Geometry check sheet. Reference: the model listing, model coordinates, mm. Face numbers are marked on the shaded views. A direction names the side the tool comes from. Coordinates: 2 decimals unless noted, no trailing zeros. Loops run counter-clockwise (first coordinate to the right, second up) from the corner with the lowest first, then second, coordinate; pieces in that order, holes last. Notation, with made-up numbers: (-9.5, 55.5) - (8.5, 55.5) arc R34 cw to (8.5, 85.5) - close; hole circle Ø5 at (34.25, -25). An arc over 180 degrees is marked (long way). One line per item, written item: value.
from build123d import *

# Parameters (mm, degrees)
SKETCH1_W                = 18.66
SKETCH1_H                = 2.314
BOSS_EXTRUDE1_DEPTH      = 2.6
BOSS_EXTRUDE2_DEPTH      = 3.91
BOSS_EXTRUDE2_DEPTH_BACK = 10.37
SKETCH2_R                = 0.33


with BuildPart() as part:
    # Sketch1 → Boss-Extrude1 (new body)
    with BuildSketch(Plane(origin=(0, 0, 0), x_dir=(1, 0, 0), z_dir=(0, 1, 0))):
        with Locations((9.33, 1.157)):
            Rectangle(SKETCH1_W, SKETCH1_H)
    extrude(amount=BOSS_EXTRUDE1_DEPTH)

    # Sketch2 → Boss-Extrude2 (add, two sides: drawn at the far end of the back side and taken through both)
    with BuildSketch(Plane(origin=(0, 2.6, 0), x_dir=(1, 0, 0), z_dir=(0, 1, 0)).offset(-BOSS_EXTRUDE2_DEPTH_BACK)):
        with Locations(Location((1.33, 1.157, 0), (0, 0, 270))):
            Circle(SKETCH2_R)
        with Locations(Location((3.11, 1.157, 0), (0, 0, 270))):
            Circle(SKETCH2_R)
        with Locations(Location((4.89, 1.157, 0), (0, 0, 270))):
            Circle(SKETCH2_R)
        with Locations(Location((6.67, 1.157, 0), (0, 0, 270))):
            Circle(SKETCH2_R)
        with Locations(Location((8.45, 1.157, 0), (0, 0, 270))):
            Circle(SKETCH2_R)
        with Locations(Location((10.23, 1.157, 0), (0, 0, 270))):
            Circle(SKETCH2_R)
        with Locations(Location((12.01, 1.157, 0), (0, 0, 270))):
            Circle(SKETCH2_R)
        with Locations(Location((13.79, 1.157, 0), (0, 0, 270))):
            Circle(SKETCH2_R)
        with Locations(Location((15.57, 1.157, 0), (0, 0, 270))):
            Circle(SKETCH2_R)
        with Locations(Location((17.35, 1.157, 0), (0, 0, 270))):
            Circle(SKETCH2_R)
    extrude(amount=BOSS_EXTRUDE2_DEPTH + BOSS_EXTRUDE2_DEPTH_BACK)


solid = part.part
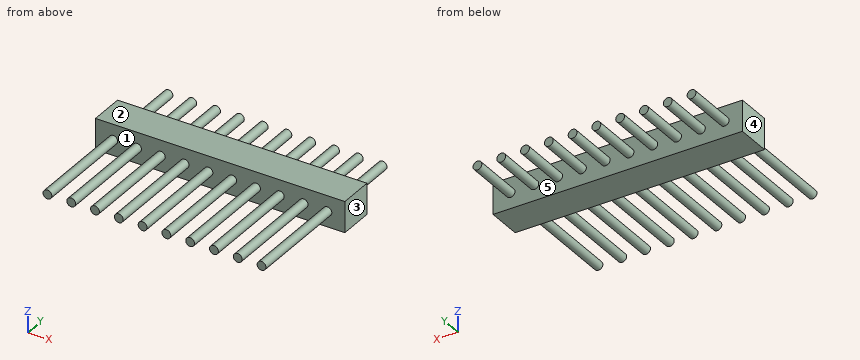
(1) Go/stop test with flat-tipped pins: pin 1 Ø3 at (x, y) = (14, -1) entering from -Z; pin 2 Ø1.5 at (x, y) = (11.5, 3.5) entering from +Z. Record where each tip stops, or that it passes through.
Reply:
pin 1: z = -2.31
pin 2: z = -0.83
(2) Material ranges on probe 1 along Y at (x, z) = (10.75, -0.1); probe 2 along Z at (x, y) = (14, -6.75); probe 3 along Z at (x, y) = (15.5, -0.5), recorded low to high. Write a range as from..to.
Reply:
probe 1: 0..2.6
probe 2: -1.41..-0.9
probe 3: -1.48..-0.83
(3) Access from +Z, -Z, +X, -X, +Y, -Y to the whole of each face (thin tool, end or side, straight path). Record for the marked faces 1 and 2.
Reply:
face 1: -Y
face 2: +Z, +X, -X, +Y, -Y
(4) Cross-section at B-B on x = 4.89. Record the cut outline in (y, z).
Reply:
outline: (-7.77, -1.49) - (0, -1.49) - (0, -2.31) - (2.6, -2.31) - (2.6, -1.49) - (6.51, -1.49) - (6.51, -0.83) - (2.6, -0.83) - (2.6, 0) - (0, 0) - (0, -0.83) - (-7.77, -0.83) - close
(5) Release check for a two-part mould opening along X. For the marked faces 3, 4 and 5 record: pulls with the +X half, pulls with the -X half, needs draft (parallel to the pull), parting line crosses it, or undercut.
Reply:
face 3: pulls with the +X half
face 4: pulls with the -X half
face 5: undercut
(6) Cross-section at C-C on z = -0.2. Record the cut outline in (x, y).
Reply:
outline: (0, 0) - (18.66, 0) - (18.66, 2.6) - (0, 2.6) - close
(7) Cross-section at A-A on y = -4.5. State how many separate pieces and enclosed holes the cut face has, and give its area (3 significant figures).
Reply:
separate pieces: 10
enclosed holes: 0
area: 3.42 mm2
(8) Cross-section at D-D on x = 11.25. Record the cut outline in (y, z), and give its area (3 significant figures).
Reply:
outline: (0, -2.31) - (2.6, -2.31) - (2.6, 0) - (0, 0) - close
area: 6.02 mm2
